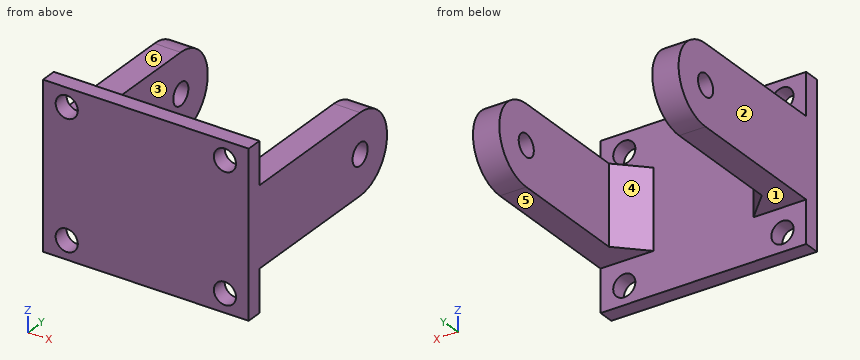
from build123d import *

# Parameters (mm, degrees)
SKETCH_1_W          = 39
SKETCH_1_H          = 31
EXTRUDE_1_DEPTH     = 3
SKETCH_5_R          = 2.1
EXTRUDE_2_DEPTH     = 5
EXTRUDE_START       = -5
SKETCH_6_R          = 2.1
EXTRUDE_3_DEPTH     = 5
SKETCH_8_R          = 2.1
CUT_EXTRUDE_1_DEPTH = 46.855752093
CHAMFER_1_SIZE      = 5


with BuildPart() as part:
    # 草图1 → 凸台-拉伸1 (new body)
    with BuildSketch(Plane(origin=(0, 0, 0), x_dir=(1, 0, 0), z_dir=(0, 1, 0))):
        Rectangle(SKETCH_1_W, SKETCH_1_H)
    extrude(amount=EXTRUDE_1_DEPTH)

    # 草图5 → 凸台-拉伸2 (add)
    with BuildSketch(Plane.ZY.offset(19.5)):
        with BuildLine():
            ThreePointArc((7.5, 31), (0, 38.5), (-7.5, 31))
            Line((-7.5, 31), (-7.5, 3))
            Line((-7.5, 3), (7.5, 3))
            Line((7.5, 3), (7.5, 31))
        make_face()
        with Locations((0, 31)):
            Circle(SKETCH_5_R, mode=Mode.SUBTRACT)
    extrude(amount=-EXTRUDE_2_DEPTH)

    # 草图6 → 凸台-拉伸3 (add)
    with BuildSketch(Plane(origin=(19.5, 0, 0), x_dir=(0, 0, -1), z_dir=(1, 0, 0)).offset(EXTRUDE_START)):
        with BuildLine():
            Line((-7.5, 31), (-7.5, 3))
            Line((-7.5, 3), (7.5, 3))
            Line((7.5, 3), (7.5, 31))
            ThreePointArc((7.5, 31), (0, 38.5), (-7.5, 31))
        make_face()
        with Locations(Location((0, 31, 0), (0, 0, 180))):
            Circle(SKETCH_6_R, mode=Mode.SUBTRACT)
    extrude(amount=EXTRUDE_3_DEPTH)

    # 草图8 → 切除-拉伸1 (cut, through all)
    with BuildSketch(Plane.XZ):
        with Locations(Location((15, 12, 0), (0, 0, 270))):
            Circle(SKETCH_8_R)
        with Locations(Location((15, -12, 0), (0, 0, 270))):
            Circle(SKETCH_8_R)
        with Locations(Location((-15, 12, 0), (0, 0, 270))):
            Circle(SKETCH_8_R)
        with Locations(Location((-15, -12, 0), (0, 0, 270))):
            Circle(SKETCH_8_R)
    extrude(amount=-CUT_EXTRUDE_1_DEPTH, mode=Mode.SUBTRACT)

    # 倒角1
    chamfer_1_edges = [part.edges().sort_by_distance(p)[0] for p in [
        (-14.5, 3, 0),
        (14.5, 3, 0),
    ]]
    chamfer(chamfer_1_edges, length=CHAMFER_1_SIZE)


solid = part.part
Here's how the part is built. I have some questions about the finished solid (model axes, mm). Face numbers are marked on the shaded views. A direction names the side the tool comes from. Give positions to 0.01 mm unless a question says otherwise; leave off trailing zeros. Order: outer loops, then holes, each group sorted by start corner. A loop starts at its lowest first (then second) coordinate and runs counter-clockwise, first axis right, second up. Notation, with made-up numbers: (54, 85) -> (104, 85) arc R23 ccw to (104, 94) -> close; hole circle Ø4 at (-21.75, 67). An arc over 180 degrees is marked (long way). One line per item, written item: value. Start each with the question number.
1. Will these pins go through, and if not, where does the flat tip stop? pin 1 Ø11 at (x, y) = (-12, 22.5) entering from -Z; pin 2 Ø5 at (y, z) = (31, 0) entering from +X; pin 3 Ø15.5 at (x, z) = (3, -0.5) entering from +Y; pin 4 Ø6 at (x, z) = (10.5, 12) entering from +Y.
2. Imagine slicing it at A-A, the plane z = 0. List the corners of the cut face in (x, y) for me.
3. Imagine slicing it at B-B, the plane y = 18.5. List the corners of the cut face in (x, z) for me.
4. For the marked faces 4, 5 and 6, which set-ups out of +Z, -Z, +X, -X, +Y, -Y let a thin tool reach every point of the face, with its end or its side?
5. I need wall thicknesses on probe 1 along X at (y, z) = (0.9, 12); probe 2 along X at (y, z) = (36, -5); probe 3 along Y at (x, z) = (18, 0). Which ranges of each line are inside material? Lowest first, please. Write a range as from..to.
6. Imagine slicing it at C-C, the plane z = 13.5. List the corners of the cut face in (x, y) for me.
7. Imagine slicing it at D-D, the plane x = -2. List the corners of the cut face in (y, z) for me.
8. We'd pull the mould along X, two halves only. Please class the marked faces 1, 2 and 3: released by +X, released by -X, zero draft, split by the parting line, or undercut.
Values follow:
1. pin 1: stops at z = -7.5
1. pin 2: stops at x = 19.5
1. pin 3: stops at y = 4.25
1. pin 4: stops at y = 3
2. outline: (-19.5, 0) -> (19.5, 0) -> (19.5, 28.9) -> (14.5, 28.9) -> (14.5, 8) -> (9.5, 3) -> (-9.5, 3) -> (-14.5, 8) -> (-14.5, 28.9) -> (-19.5, 28.9) -> close; (-19.5, 33.1) -> (-14.5, 33.1) -> (-14.5, 38.5) -> (-19.5, 38.5) -> close; (14.5, 33.1) -> (19.5, 33.1) -> (19.5, 38.5) -> (14.5, 38.5) -> close
3. outline: (-19.5, -7.5) -> (-14.5, -7.5) -> (-14.5, 7.5) -> (-19.5, 7.5) -> close; (14.5, -7.5) -> (19.5, -7.5) -> (19.5, 7.5) -> (14.5, 7.5) -> close
4. face 4: +Z, -Z, +Y
4. face 5: -Z, +X, -X, +Y
4. face 6: +Z, +X, -X, +Y
5. probe 1: x = -19.5..-17.1, -12.9..12.9, 17.1..19.5
5. probe 2: x = -19.5..-14.5, 14.5..19.5
5. probe 3: y = 0..28.9, 33.1..38.5
6. outline: (-19.5, 0) -> (-16.47, 0) -> (-16.47, 3) -> (-19.5, 3) -> close; (-13.53, 0) -> (13.53, 0) -> (13.53, 3) -> (-13.53, 3) -> close; (16.47, 0) -> (19.5, 0) -> (19.5, 3) -> (16.47, 3) -> close
7. outline: (0, -15.5) -> (3, -15.5) -> (3, 15.5) -> (0, 15.5) -> close
8. face 1: zero draft
8. face 2: released by -X
8. face 3: undercut
